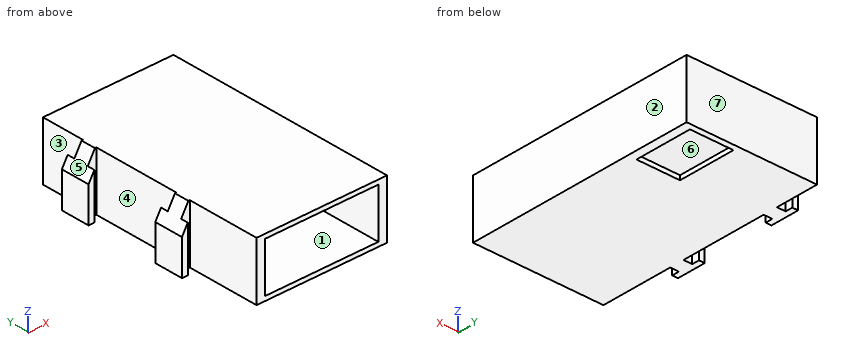
Autodesk Inventor part; units mm, degrees
ref_plane "作業平面1" through (0, 45, 0) normal (0, 1, 0) x (1, 0, 0)
ref_plane "作業平面2" through (0, 80, 0) normal (0, -1, 0) x (1, 0, 0)
ref_plane "YZ Plane" through (0, 0, 0) normal (1, 0, 0) x (0, 1, 0)
sketch "スケッチ1" plane through (0, 0, 0) normal (0, 1, 0) x (-1, 0, 0)
  line L0 (-22.5, -10) -> (22.5, -10)
  line L1 (22.5, -10) -> (22.5, 10)
  line L2 (22.5, 10) -> (-22.5, 10)
  line L3 (-22.5, 10) -> (-22.5, -10)
  line L4 (-22.5, -10) -> (22.5, 10) construction
  line L5 (22.5, -10) -> (-22.5, 10) construction
  point P0 (0, 0)
  dimension "d0" = 45
  dimension "d1" = 20
extrude "押し出し1" add sketch "スケッチ1" along normal blind 90
sketch "スケッチ2" plane through (-22.5, 0, 10) normal (0, 0, 1) x (1, 0, 0)
  line L0 (0, 0) -> (0, 90)
  line L1 (0, 65) -> (-3, 65)
  line L2 (-3, 65) -> (-3, 60)
  line L3 (-3, 60) -> (0, 60)
  line L4 (0, 60) -> (0, 65)
  line L5 (-3, 67.5) -> (-5, 67.5)
  line L6 (-5, 67.5) -> (-5, 57.5)
  line L7 (-5, 57.5) -> (-3, 57.5)
  line L8 (-3, 57.5) -> (-3, 67.5)
  line L9 (0, 90) -> (45, 90)
  point P0 (22.5, 0)
  point P1 (-5, 62.5)
  point P2 (-3, 62.5)
  point P3 (-3, 60)
  point P4 (0, 60)
  point P5 (-3, 65)
  dimension "d14" = 5
  dimension "d15" = 10
  dimension "d16" = 2
  dimension "d17" = 3
  dimension "d18" = 25
ref_plane "作業平面1" through (0, 45, 0) normal (0, 1, 0) x (1, 0, 0)
extrude "押し出し2" add sketch "スケッチ2" against normal up to surface (20 mm away)
mirror "ミラー1" about plane through (0, 45, 0) normal (0, 1, 0) of "押し出し2"
sketch "スケッチ3" plane through (-27.5, 67.5, 10) normal (0, 1, 0) x (1, 0, 0)
  line L0 (4.5, 0) -> (-25.5, 51.9615)
  line L1 (2, 20) -> (0, 20)
  line L2 (0, 0) -> (0, 20)
  line L3 (2, 0) -> (0, 0)
  line L4 (2, 0) -> (2, 20)
  line L5 (5, 20) -> (2, 20)
  line L6 (2, 0) -> (2, 20)
  line L7 (5, 0) -> (2, 0)
  line L8 (5, 20) -> (5, 0)
  point P0 (27.5, 10)
  point P1 (4.5, 0)
  point P2 (0, 7.7942)
extrude "押し出し3" cut sketch "スケッチ3" against normal through all contours L7 L4 L0 | L4 L3 L2 L0
sketch "スケッチ4" plane through (22.5, 0, 10) normal (1, 0, 0) x (0, 0, -1)
  line L0 (6.75, 92.2249) -> (6.75, 87.9989)
  line L1 (6.75, 87.9989) -> (1.25, 90.7989)
  line L2 (1.25, 92.2249) -> (1.25, 90.7989)
  line L3 (20, 90) -> (0, 90)
  line L4 (6.95, 90) -> (6.95, 87.7989)
  line L5 (6.95, 87.7989) -> (0, 87.7989)
  line L6 (0, 0) -> (0, 90)
  line L7 (0, 90) -> (20, 90)
  arc A0 (7.95, 90) -> (20, 90.2989) centre (12.7443, 139.7696) ccw
  line L8 (20, 0) -> (20, 90)
  point P0 (10, 0)
  point P1 (7.95, 90)
  point P2 (17.5386, 90)
  dimension "d26" = 0.2
  dimension "d27" = 0.2
  dimension "d28" = 50
  dimension "d29" = 1
  dimension "d32" = 2.5
extrude "押し出し4" cut sketch "スケッチ4" against normal through all
sketch "スケッチ5" plane through (22.5, 87.7989, 3.05) normal (0, 0, 1) x (1, 0, 0)
  line L0 (-36.25, 2.2011) -> (-36.25, 5.1444)
  line L1 (-30.25, 3.7011) -> (-30.25, 2.2011)
  line L2 (-24.85, 7.7011) -> (-24.85, 2.2011)
  line L3 (-20.65, 2.2011) -> (-20.65, 7.7011)
  line L4 (-24.85, 7.7011) -> (-24.85, 2.2011)
  line L5 (-15.25, 2.2011) -> (-15.25, 3.7011)
  line L6 (-9.25, 9.2011) -> (-9.25, 6.2579)
  line L7 (0, 0) -> (-45, 0)
  line L8 (-36.25, 2.2011) -> (-45, 2.2011)
  line L9 (-45, 2.2011) -> (-45, 0)
  line L10 (-45, 0) -> (-36.25, 0)
  line L11 (-36.25, 0) -> (-36.25, 2.2011)
  line L12 (-30.25, 2.2011) -> (-24.85, 2.2011)
  line L13 (-24.85, 2.2011) -> (-24.85, 0)
  line L14 (-24.85, 0) -> (-30.25, 0)
  line L15 (-30.25, 0) -> (-30.25, 2.2011)
  line L16 (-20.65, 2.2011) -> (-15.25, 2.2011)
  line L17 (-15.25, 2.2011) -> (-15.25, 0)
  line L18 (-15.25, 0) -> (-20.65, 0)
  line L19 (-20.65, 0) -> (-20.65, 2.2011)
  line L20 (-9.25, 6.2579) -> (0, 6.2579)
  line L21 (0, 6.2579) -> (0, 0)
  line L22 (0, 0) -> (-9.25, 0)
  line L23 (-9.25, 0) -> (-9.25, 6.2579)
  point P0 (-22.5, -87.7989)
  point P1 (-9.25, 0)
extrude "押し出し5" add sketch "スケッチ5" along normal up to surface (6.95 mm away)
sketch "スケッチ6" plane through (0, 0, 0) normal (0, -1, 0) x (1, 0, 0)
  line L0 (19.5, -8.5) -> (-19.5, -8.5)
  line L1 (-19.5, -8.5) -> (-19.5, 8.5)
  line L2 (-19.5, 8.5) -> (19.5, 8.5)
  line L3 (19.5, 8.5) -> (19.5, -8.5)
  line L4 (19.5, -8.5) -> (-19.5, 8.5) construction
  line L5 (-19.5, -8.5) -> (19.5, 8.5) construction
  point P0 (0, 0)
  dimension "d35" = 39
  dimension "d36" = 17
extrude "押し出し6" cut sketch "スケッチ6" against normal blind 78
sketch "スケッチ7" plane through (-19.5, 0, -8.5) normal (0, 0, 1) x (1, 0, 0)
  line L0 (39, 0) -> (0, 0)
  line L1 (39, 0) -> (39, 78)
  line L2 (39, 78) -> (0, 78)
  line L3 (0, 0) -> (0, 78)
  line L4 (39, 78) -> (24, 78)
  line L5 (24, 78) -> (24, 58)
  line L6 (24, 58) -> (39, 58)
  line L7 (39, 58) -> (39, 78)
  point P0 (19.5, 0)
  dimension "d39" = 15
  dimension "d40" = 20
extrude "押し出し7" cut sketch "スケッチ7" against normal through all contours L6 L5 L2 L1
sketch "スケッチ8" plane through (13.25, 94.0568, 3.05) normal (0, 1, 0) x (1, 0, 0)
  line L0 (9.25, 0) -> (9.25, -6.95)
  line L1 (9.25, -6.95) -> (-35.75, -6.95)
  line L2 (-35.75, -6.95) -> (-35.75, 13.05)
  line L3 (-35.75, 13.05) -> (9.25, 13.05)
  line L4 (9.25, 13.05) -> (9.25, -6.95)
  point P0 (-13.25, 3.05)
ref_plane "作業平面2" through (0, 80, 0) normal (0, -1, 0) x (1, 0, 0)
extrude "押し出し8" cut sketch "スケッチ8" against normal up to surface (14.0568 mm away)
equation "\"d27\" = d26"
properties part number "battery"
Input: part model. Units: mm. Frame: model coordinates. Face numbers are marked on the shaded views. A direction names the side the tool comes from. Give positions to 0.01 mm unless a question says otherwise; leave off trailing zeros. Order: outer loops, then holes, each group sorted by start corner. A loop starts at its lowest first (then second) coordinate and runs counter-clockwise, first axis right, second up. Notation, with made-up numbers: (-22, 17.25) - (-8, 17.25) arc R16 cw to (-8, 33.25) - close; hole circle Ø3 at (22.5, 82.25). An arc over 180 degrees is marked (long way). One line per item, written item: value.
1. Reachability of the marked faces 1, 2, 3 and 4 from +Z, -Z, +X, -X, +Y, -Y: full face, straight path, thin tool, end or side. Return the list, or none.
Determined:
face 1: -Y
face 2: +Z, -Z, +X, +Y, -Y
face 3: +Z, -Z, +Y
face 4: +Z, -Z
2. Cut plane B-B, the plane y = 6. Output: boundary loops of the cut face in (x, z).
Determined:
outline: (-22.5, -10) - (22.5, -10) - (22.5, 10) - (-22.5, 10) - close; hole (-19.5, -8.5) - (19.5, -8.5) - (19.5, 8.5) - (-19.5, 8.5) - close
3. Cut plane A-A, the plane x = 11.5. Output: boundary loops of the cut face in (y, z), and give its area (3 significant figures).
Determined:
outline: (0, -10) - (58, -10) - (58, -8.5) - (0, -8.5) - close; (0, 8.5) - (78, 8.5) - (78, -10) - (80, -10) - (80, 10) - (0, 10) - close
area: 244 mm2
4. Draft query along X for the marked faces 5, 6 and 7. Return one class per face: released by +X, released by -X, zero draft, split by the parting line, or undercut.
Determined:
face 5: released by -X
face 6: undercut
face 7: zero draft
5. Cut plane C-C, the plane z = -0.5. Output: boundary loops of the cut face in (x, y).
Determined:
outline: (-27.5, 22.5) - (-25.5, 22.5) - (-25.5, 25) - (-22.5, 25) - (-22.5, 0) - (-19.5, 0) - (-19.5, 78) - (19.5, 78) - (19.5, 0) - (22.5, 0) - (22.5, 80) - (-22.5, 80) - (-22.5, 65) - (-25.5, 65) - (-25.5, 67.5) - (-27.5, 67.5) - (-27.5, 57.5) - (-25.5, 57.5) - (-25.5, 60) - (-22.5, 60) - (-22.5, 30) - (-25.5, 30) - (-25.5, 32.5) - (-27.5, 32.5) - close
6. Pin query (flat end, axial travel): pin 1 Ø0.9 at (x, z) = (-24.5, -0.5) entering from +Y; pin 2 Ø5.5 at (y, z) = (54, 1) entering from -X; pin 3 Ø2.5 at (x, z) = (-24.5, 4) entering from -Y. Return the tip coordinate at first contact, or that it passes through.
Determined:
pin 1: y = 65
pin 2: x = -22.5
pin 3: y = 22.5
7. Cut plane D-D, the plane y = 71.5. Output: boundary loops of the cut face in (x, z).
Determined:
outline: (-22.5, -10) - (4.5, -10) - (4.5, -8.5) - (-19.5, -8.5) - (-19.5, 8.5) - (19.5, 8.5) - (19.5, -10) - (22.5, -10) - (22.5, 10) - (-22.5, 10) - close
8. Line query: probe 1 along Z at (x, y) = (-15, 55); probe 2 along X at (y, z) = (21.5, 3.75); probe 3 along Y at (x, z) = (12, -8.75). Output: solid intervals per line, ascending.
Determined:
probe 1: -10 to -8.5, 8.5 to 10
probe 2: -22.5 to -19.5, 19.5 to 22.5
probe 3: 0 to 58, 78 to 80
